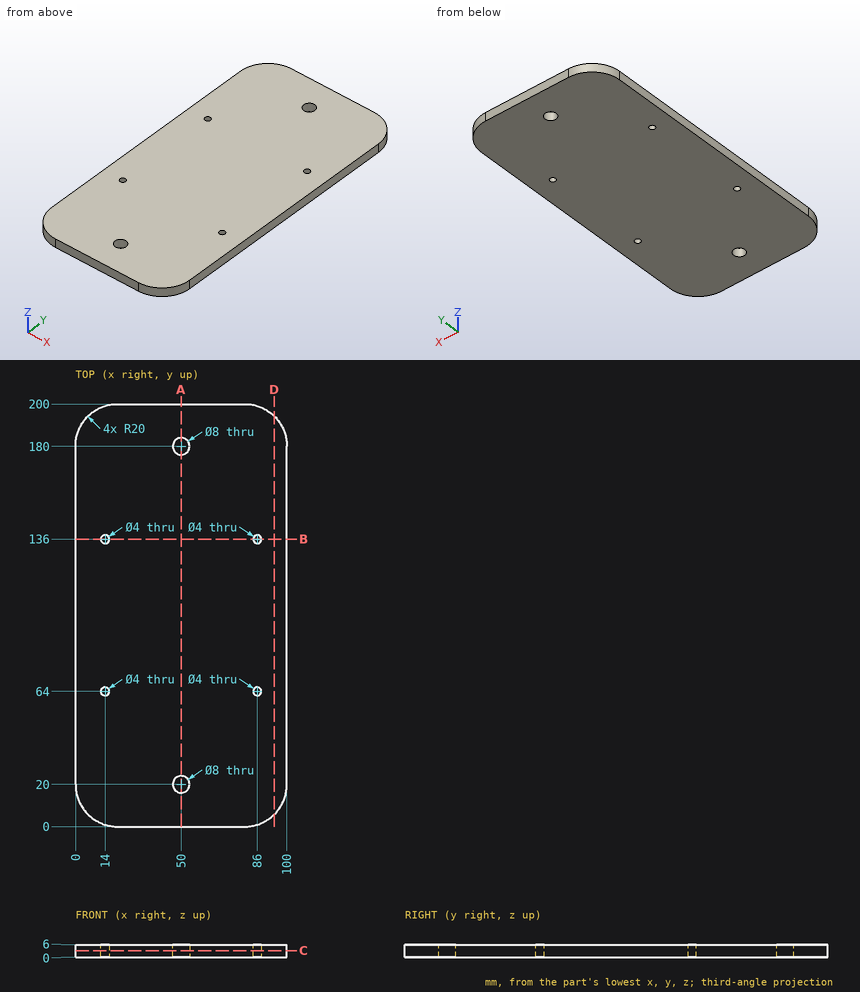
Here's the drawing with two shaded views (mm, measured from the low corner). I have some questions. Give positions to 0.01 mm unless a question says otherwise; leave off trailing zeros. Loops run counter-clockwise (first coordinate to the right, second up) from the corner with the lowest first, then second, coordinate; pieces in that order, holes last. Notation, with made-up numbers: (10, 76) -> (59, 76) arc R13 cw to (59, 98) -> close; hole circle Ø11 at (32.25, 70). An arc over 180 degrees is marked (long way). Answer as a JSON object with one key per item and string values. Group by question number.
Item 1: I need wall thicknesses on L1, parallel to Y at x = 49.5, z = 3.9; L2, parallel to Y at x = 14, z = 3.05; L3, parallel to Y at x = 90, z = 2. Which ranges of each line are inside material? Lowest first, please.
Item 2: Imagine slicing it at D-D on x = 94. Write out the boundary of the cut face in (y, z).
Item 3: Imagine slicing it at A-A on x = 50. Write out the boundary of the cut face in (y, z).
Item 4: Imagine slicing it at B-B on y = 136. Write out the boundary of the cut face in (x, z), then the cut area to 3 significant figures.
Item 5: Imagine slicing it at C-C on z = 3.2. Write out the boundary of the cut face in (x, y).
Answer list:
{
 "1": {"L1": "y = 0 to 16.03, 23.97 to 176.03, 183.97 to 200", "L2": "y = 0.92 to 62, 66 to 134, 138 to 199.08", "L3": "y = 2.68 to 197.32"},
 "2": {"outline": "(5.72, 0) -> (194.28, 0) -> (194.28, 6) -> (5.72, 6) -> close"},
 "3": {"outline": "(0, 0) -> (16, 0) -> (16, 6) -> (0, 6) -> close; (24, 0) -> (176, 0) -> (176, 6) -> (24, 6) -> close; (184, 0) -> (200, 0) -> (200, 6) -> (184, 6) -> close"},
 "4": {"outline": "(0, 0) -> (12, 0) -> (12, 6) -> (0, 6) -> close; (16, 0) -> (84, 0) -> (84, 6) -> (16, 6) -> close; (88, 0) -> (100, 0) -> (100, 6) -> (88, 6) -> close", "area": "552 mm2"},
 "5": {"outline": "(0, 20) arc R20 ccw to (20, 0) -> (80, 0) arc R20 ccw to (100, 20) -> (100, 180) arc R20 ccw to (80, 200) -> (20, 200) arc R20 ccw to (0, 180) -> close; hole circle Ø4 at (14, 64); hole circle Ø4 at (14, 136); hole circle Ø8 at (50, 20); hole circle Ø8 at (50, 180); hole circle Ø4 at (86, 64); hole circle Ø4 at (86, 136)"}
}
